Source: CAD feature listing. Evaluate the final solid. Frame: model axes, mm. A direction names the side the tool comes from. Give positions to 0.01 mm unless a question says otherwise; leave off trailing zeros. Write each loop counter-clockwise with the first axis right and the second up, starting at its lowest first coordinate (ties: lowest second). Pieces come first, ordered by that corner, then holes. Notation, with made-up numbers: (3.25, 24) -> (8.25, 24) arc R21 ccw to (8.25, 42) -> close; hole circle Ø5 at (61.25, 63.25). An arc over 180 degrees is marked (long way). Write item = value, one per line.
from build123d import *

# Parameters (mm, degrees)
SKETCH2_W           = 50
SKETCH2_H           = 20
BOSS_EXTRUDE1_DEPTH = 3
FILLET1_R           = 10


with BuildPart() as part:
    # Sketch2 → Boss-Extrude1 (new body)
    with BuildSketch(Plane.XY):
        Rectangle(SKETCH2_W, SKETCH2_H)
        with BuildLine():
            Line((-15, 2.5), (15, 2.5))
            ThreePointArc((15, 2.5), (17.5, 0), (15, -2.5))
            Line((15, -2.5), (-15, -2.5))
            ThreePointArc((-15, -2.5), (-17.5, 0), (-15, 2.5))
        make_face(mode=Mode.SUBTRACT)
    extrude(amount=BOSS_EXTRUDE1_DEPTH)

    # Fillet1
    fillet1_edges = [part.edges().sort_by_distance(p)[0] for p in [
        (25, -10, 1.5),
        (-25, -10, 1.5),
        (-25, 10, 1.5),
        (25, 10, 1.5),
    ]]
    fillet(fillet1_edges, radius=FILLET1_R - 0.0001)  # a hair under: the kernel refuses the full size


solid = part.part
(1) Section query C-C (y = 4.25). Return loops of the section in (x, z), plus the area to 3 significant figures.
Values follow:
outline = (-24.05, 0) -> (24.05, 0) -> (24.05, 3) -> (-24.05, 3) -> close
area = 144 mm2
(2) Pull-direction query (X, two-part tool) for faces 1 (the face through (0, 10, 1)), 2 (the face through (21.99, 7.15, 1.52)), 3 (the face through (0, -2.5, 1)); classes: pulls with the +X half, pulls with the -X half, needs draft (parallel to the pull), parting line crosses it, or undercut.
Values follow:
face_1 = needs draft
face_2 = pulls with the +X half
face_3 = undercut
(3) Section query B-B (x = 3.5). Return loops of the section in (y, z), plus the area to 3 significant figures.
Values follow:
outline = (-10, 0) -> (-2.5, 0) -> (-2.5, 3) -> (-10, 3) -> close; (2.5, 0) -> (10, 0) -> (10, 3) -> (2.5, 3) -> close
area = 45.0 mm2
(4) Section query D-D (x = -17). Return loops of the section in (y, z).
Values follow:
outline = (-9.8, 0) -> (-1.5, 0) -> (-1.5, 3) -> (-9.8, 3) -> close; (1.5, 0) -> (9.8, 0) -> (9.8, 3) -> (1.5, 3) -> close
(5) Material intervals for line 1 (Y direction, x = -1.5, z = 0.2); line 2 (X direction, y = -0.25, z = 1.7); line 3 (X direction, y = -0.5, z = 1.3), sorted ascending.
Values follow:
line_1 = -10 to -2.5, 2.5 to 10
line_2 = -25 to -17.49, 17.49 to 25
line_3 = -24.99 to -17.45, 17.45 to 24.99
(6) Access query for faces 4 (the face through (17.5, 0.1, 1.5)), 5 (the face through (-22.15, 6.99, 1.52)). Directions: +Z, -Z, +X, -X, +Y, -Y. A direction counts if a zero-diameter tool reaches every point of the face in a straight line with its end or side. Return the directions, or none.
Values follow:
face_4 = +Z, -Z
face_5 = +Z, -Z, -X, +Y
